from build123d import *

# Parameters (mm, degrees)
SKETCH_W   = 180
SKETCH_H   = 60
SKETCH_R   = 2.5
SKETCH_W_2 = 17
SKETCH_H_2 = 30
PAD_DEPTH  = 3


with BuildPart() as part:
    # Sketch → Pad (new body)
    with BuildSketch(Plane.XY):
        with Locations((90, 30)):
            Rectangle(SKETCH_W, SKETCH_H)
        with Locations((10, 55)):
            Circle(SKETCH_R, mode=Mode.SUBTRACT)
        with Locations((170, 55)):
            Circle(SKETCH_R, mode=Mode.SUBTRACT)
        with Locations((170, 5)):
            Circle(SKETCH_R, mode=Mode.SUBTRACT)
        with Locations((10, 5)):
            Circle(SKETCH_R, mode=Mode.SUBTRACT)
        with Locations((11.5, 30)):
            Rectangle(SKETCH_W_2, SKETCH_H_2, mode=Mode.SUBTRACT)
        with Locations((168.5, 30)):
            Rectangle(SKETCH_W_2, SKETCH_H_2, mode=Mode.SUBTRACT)
    extrude(amount=PAD_DEPTH)


solid = part.part
Check sheet for the modelled part. Datum: model origin and axes. Units: mm. A direction names the side the tool comes from. Coordinates: 2 decimals unless noted, no trailing zeros. Write each loop counter-clockwise with the first axis right and the second up, starting at its lowest first coordinate (ties: lowest second). Pieces come first, ordered by that corner, then holes.
Item 1: Depth check by flat-ended pin: pin 1 Ø3 at (x, y) = (80.5, 8) entering from -Z; pin 2 Ø3 at (x, y) = (10, 5) entering from -Z. Enter the tip coordinate at first touch or a pass-through.
Numbers:
pin 1: stops at z = 0
pin 2: passes through
Item 2: Cross-section at A-A on y = 5. Record the boundary of the cut face in (x, z).
Numbers:
outline: (0, 0) - (7.5, 0) - (7.5, 3) - (0, 3) - close; (12.5, 0) - (167.5, 0) - (167.5, 3) - (12.5, 3) - close; (172.5, 0) - (180, 0) - (180, 3) - (172.5, 3) - close
Item 3: Cross-section at B-B on x = 10. Record the boundary of the cut face in (y, z).
Numbers:
outline: (0, 0) - (2.5, 0) - (2.5, 3) - (0, 3) - close; (7.5, 0) - (15, 0) - (15, 3) - (7.5, 3) - close; (45, 0) - (52.5, 0) - (52.5, 3) - (45, 3) - close; (57.5, 0) - (60, 0) - (60, 3) - (57.5, 3) - close
Item 4: Cross-section at C-C on z = 1.9. Record the boundary of the cut face in (x, y).
Numbers:
outline: (0, 0) - (180, 0) - (180, 60) - (0, 60) - close; hole (3, 15) - (20, 15) - (20, 45) - (3, 45) - close; hole circle Ø5 at (10, 5); hole circle Ø5 at (10, 55); hole (160, 15) - (177, 15) - (177, 45) - (160, 45) - close; hole circle Ø5 at (170, 5); hole circle Ø5 at (170, 55)
Item 5: Scan lines: probe 1 along X at (y, z) = (39, 1.95); probe 2 along Y at (x, z) = (170, 1); probe 3 along Y at (x, z) = (13.5, 0.5). Record each from-to range of solid material in increasing order.
Numbers:
probe 1: x = 0 to 3, 20 to 160, 177 to 180
probe 2: y = 0 to 2.5, 7.5 to 15, 45 to 52.5, 57.5 to 60
probe 3: y = 0 to 15, 45 to 60
Item 6: Mould release check, pull along Y, two halves, no side actions. Record for faces 1 (the face through (172.385, 55.751, 1.479)), 2 (the face through (89, 0, 1)), 3 (the face through (0, 30, 1)): released by +Y, released by -Y, zero draft, split by the parting line, or undercut.
Numbers:
face 1: undercut
face 2: released by -Y
face 3: zero draft
Item 7: Cross-section at D-D on y = 18. Record the boundary of the cut face in (x, z), then the cut area to 3 significant figures.
Numbers:
outline: (0, 0) - (3, 0) - (3, 3) - (0, 3) - close; (20, 0) - (160, 0) - (160, 3) - (20, 3) - close; (177, 0) - (180, 0) - (180, 3) - (177, 3) - close
area: 438 mm2
Item 8: Access from +Z, -Z, +X, -X, +Y, -Y to the whole of each face (thin tool, end or side, straight path). Record for faces 4 (the face through (20, 30, 1)), 5 (the face through (89, 30, 0)).
Numbers:
face 4: +Z, -Z
face 5: -Z, +X, -X, +Y, -Y
